Could you check a few things on this model? Use its own coordinates, in mm. Face numbers are marked on the shaded views. A direction names the side the tool comes from. Coordinates: 2 decimals unless noted, no trailing zeros. Loops run counter-clockwise (first coordinate to the right, second up) from the corner with the lowest first, then second, coordinate; pieces in that order, holes last.
from build123d import *

# Parameters (mm, degrees)
SALIENTE_EXTRUIR2_DEPTH = 3.2


with BuildPart() as part:
    # Croquis1 → Saliente-Extruir2 (new body)
    with BuildSketch(Plane(origin=(0, 0, 0), x_dir=(1, 0, 0), z_dir=(0, 1, 0))):
        with BuildLine():
            Line((10, 21.5), (7, 21.5))
            Line((7, 21.5), (7, 20.1))
            Line((7, 20.1), (3, 20.1))
            Line((3, 20.1), (3, 21.5))
            Line((3, 21.5), (0, 21.5))
            Line((0, 21.5), (0, 15.6))
            Line((0, 15.6), (-3, 15.6))
            Line((-3, 15.6), (-3, 9.6))
            Line((-3, 9.6), (0, 9.6))
            Line((0, 9.6), (0, 0))
            Line((0, 0), (0.171572875, 0))
            ThreePointArc((0.171572875, 0), (1.319623172, 0.228361402), (2.292893219, 0.878679656))
            Line((2.292893219, 0.878679656), (47.121320344, 45.707106781))
            ThreePointArc((47.121320344, 45.707106781), (47.771638598, 46.680376828), (48, 47.828427125))
            Line((48, 47.828427125), (48, 48))
            Line((48, 48), (38.4, 48))
            Line((38.4, 48), (38.4, 51))
            Line((38.4, 51), (32.4, 51))
            Line((32.4, 51), (32.4, 48))
            Line((32.4, 48), (26.5, 48))
            Line((26.5, 48), (26.5, 45))
            Line((26.5, 45), (27.9, 45))
            Line((27.9, 45), (27.9, 41))
            Line((27.9, 41), (26.5, 41))
            Line((26.5, 41), (26.5, 38))
            Line((26.5, 38), (23.3, 38))
            Line((23.3, 38), (23.3, 41))
            Line((23.3, 41), (21.9, 41))
            Line((21.9, 41), (21.9, 45))
            Line((21.9, 45), (23.3, 45))
            Line((23.3, 45), (23.3, 48))
            Line((23.3, 48), (17.4, 48))
            Line((17.4, 48), (17.4, 51))
            Line((17.4, 51), (11.4, 51))
            Line((11.4, 51), (11.4, 48))
            Line((11.4, 48), (0, 48))
            Line((0, 48), (0, 36.6))
            Line((0, 36.6), (-3, 36.6))
            Line((-3, 36.6), (-3, 30.6))
            Line((-3, 30.6), (0, 30.6))
            Line((0, 30.6), (0, 24.7))
            Line((0, 24.7), (3, 24.7))
            Line((3, 24.7), (3, 26.1))
            Line((3, 26.1), (7, 26.1))
            Line((7, 26.1), (7, 24.7))
            Line((7, 24.7), (10, 24.7))
            Line((10, 24.7), (10, 21.5))
        make_face()
    extrude(amount=SALIENTE_EXTRUIR2_DEPTH)


solid = part.part
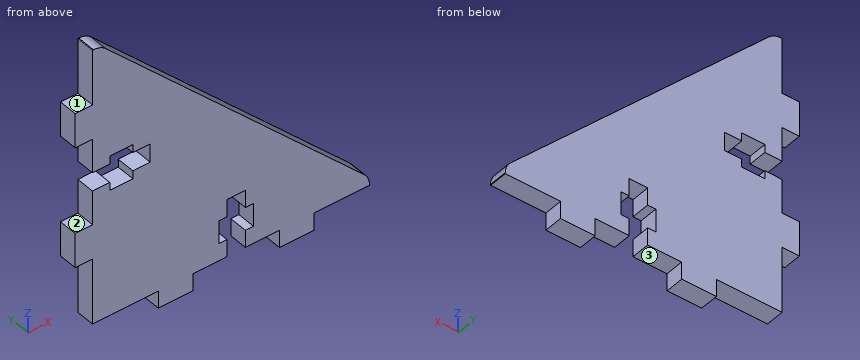
(1) Imagine slicing it at A-A, the plane x = 16. Write out the boundary of the cut face in (y, z), and give its area (3 significant figures).
Answers:
outline: (0, -51) - (3.2, -51) - (3.2, -14.59) - (0, -14.59) - close
area: 117 mm2
(2) For pin 1 (1 mm diameter, centred on y = 1, z = -43.5, fed in from -X); pin 2 (0.9 mm diameter, centred on y = 1, z = -50, fed in from -X); pin 3 (2 mm diameter, centred on x = 4, z = -35.5, fed in from -Y); pin 4 (0.9 mm diameter, centred on x = -2, y = 1, fed in from -Z), each with a flat end and sliding along its axis, tell me the tip position at first contact or that it passes through.
Answers:
pin 1: stops at x = 0
pin 2: stops at x = 11.4
pin 3: stops at y = 0
pin 4: stops at z = -36.6
(3) Which directions (+Z, -Z, +X, -X, +Y, -Y) give clear straight access to the entire face, cutting with the end or side of a thin tool? Please do the marked faces 1, 2 and 3.
Answers:
face 1: +Z, -X, +Y, -Y
face 2: -X, +Y, -Y
face 3: -Z, +Y, -Y
(4) I need wall thicknesses on probe 1 along Z at (x, y) = (-0.5, 2.05); probe 2 along Z at (x, y) = (21.5, 1.8); probe 3 along X at (y, z) = (2.65, -40). Which ranges of each line are inside material? Lowest first, please.
Answers:
probe 1: z = -36.6 to -30.6, -15.6 to -9.6
probe 2: z = -48 to -20.09
probe 3: x = 0 to 23.3, 26.5 to 41.41
(5) Imagine slicing it at B-B, the plane z = -9. Write out the boundary of the cut face in (x, y), and give its area (3 significant figures).
Answers:
outline: (0, 0) - (10.41, 0) - (10.41, 3.2) - (0, 3.2) - close
area: 33.3 mm2
